Here's the drawing with two shaded views (mm, measured from the low corner). I have some questions. A direction names the side the tool comes from. Round coordinates to 2 decimals unless told otherwise and drop trailing zeros. Order: outer loops, then holes, each group sorted by start corner. A loop starts at its lowest first (then second) coordinate and runs counter-clockwise, first axis right, second up.
Q1. For the marked faces 1 and 2, which set-ups out of +Z, -Z, +X, -X, +Y, -Y let a thin tool reach every point of the face, with its end or its side?
Q2. If we section it at B-B (x = 67): Please give me the cut outline in (y, z), plus the area to 3 significant figures.
Q3. If we section it at C-C (x = 30): Please give me the cut outline in (y, z).
Q4. If we section it at A-A (z = 40): Count the separate pieces of the cut face and the enclosed holes in it, plus the area to 3 significant figures.
Q5. If I drill on line 1 (Y direction, x = 83.55, z = 40); line 2 (Z direction, x = 81.4, y = 77.5); line 3 (Y direction, x = 11, z = 36.5), over which ranges is the centre line in solid material (lowest first)?
Q6. Will this pin go through, and if not, where does the flat tip stop? P1, Ø2, axis at y = 111, z = 37.5, coming from the -X side.
Q7. If we section it at D-D (y = 77.5): Please give me the cut outline in (x, z).
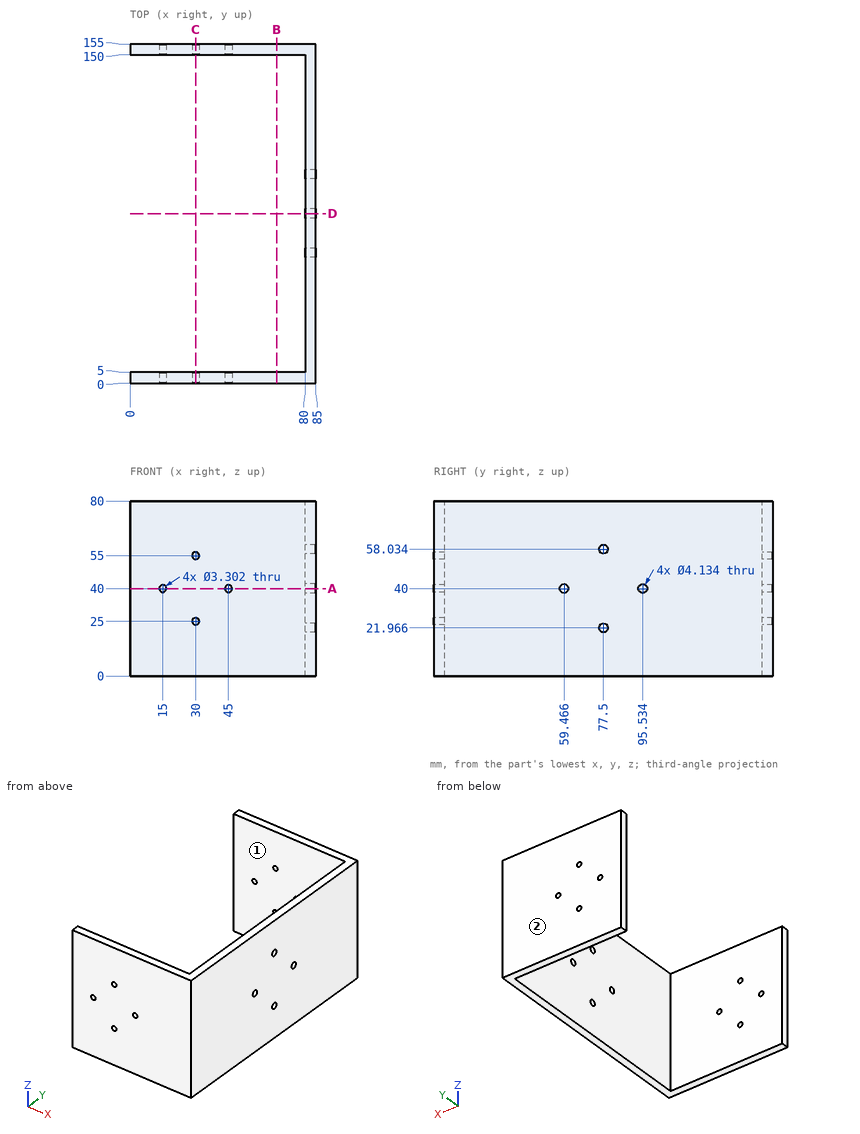
Solution:
1. face 1: +Z, -Z, -X
1. face 2: +Z, -Z, +X, -X, +Y
2. outline: (0, 0) - (5, 0) - (5, 80) - (0, 80) - close; (150, 0) - (155, 0) - (155, 80) - (150, 80) - close
2. area: 800 mm2
3. outline: (0, 0) - (5, 0) - (5, 23.35) - (0, 23.35) - close; (0, 26.65) - (5, 26.65) - (5, 53.35) - (0, 53.35) - close; (0, 56.65) - (5, 56.65) - (5, 80) - (0, 80) - close; (150, 0) - (155, 0) - (155, 23.35) - (150, 23.35) - close; (150, 26.65) - (155, 26.65) - (155, 53.35) - (150, 53.35) - close; (150, 56.65) - (155, 56.65) - (155, 80) - (150, 80) - close
4. separate pieces: 7
4. enclosed holes: 0
4. area: 1,470 mm2
5. line 1: y = 0 to 57.4, 61.53 to 93.47, 97.6 to 155
5. line 2: z = 0 to 19.9, 24.03 to 55.97, 60.1 to 80
5. line 3: y = 0 to 5, 150 to 155
6. P1: stops at x = 80
7. outline: (80, 0) - (85, 0) - (85, 19.9) - (80, 19.9) - close; (80, 24.03) - (85, 24.03) - (85, 55.97) - (80, 55.97) - close; (80, 60.1) - (85, 60.1) - (85, 80) - (80, 80) - close
